Verification items for the finished model (mm, model axes). A direction names the side the tool comes from. Coordinates: 2 decimals unless noted, no trailing zeros. Loops run counter-clockwise (first coordinate to the right, second up) from the corner with the lowest first, then second, coordinate; pieces in that order, holes last.
Q1. Access from +Z, -Z, +X, -X, +Y, -Y to the whole of each face (thin tool, end or side, straight path). Record for faces 4 (the face through (21.5, -1, -2)), 5 (the face through (0.217, -2.076, -0.203)), 6 (the face through (20.7, 1.1, -1.7)), 7 (the face through (-3, 0, 8)).
Q2. Go/stop test with flat-tipped pins: P1, Ø2, axis at y = 1, z = 0.5, coming from the +X side; P2, Ø12, axis at x = 12.5, z = 13.5, coming from the +Y side; P3, Ø1.5, axis at x = 1, y = 1, coming from the -Z side. Record where each tip stops, or that it passes through.
Q3. Material ranges on probe 1 along Z at (x, y) = (1.75, -0.8); probe 2 along X at (y, z) = (-2.4, 8.25); probe 3 along X at (y, z) = (1.95, 2.75), recorded low to high.
Q4. Sectioned sample at B-B (z = 2.75). Enter the section's corners in (x, y), then the cut area to 3 significant figures.
Q5. Sectioned sample at A-A (x = 10.75). Enter the section's corners in (y, z).
Q6. Mould release check, pull along Z, two halves, no side actions. Record for faces 1 (the face through (20.74, -0.63, -1.88)), 2 (the face through (1, 0, 0)), 3 (the face through (0, 0, 16.6)): +Z half, -Z half, draft (parallel to the pull), parting line (faces both ways), or undercut.
```python
from build123d import *

# Parameters (mm, degrees)
SKETCH1_R           = 3
CASING_DEPTH        = 16.6
CASING_CHAMFER_SIZE = 0.3
SKETCH3_R           = 1
SKETCH4_R           = 0.7
EXPOSED_WIRE_DEPTH  = 1.5


with BuildPart() as part:
    # Sketch1 → Casing (new body)
    with BuildSketch(Plane.XY):
        Circle(SKETCH1_R)
    extrude(amount=CASING_DEPTH)

    # Casing Chamfer
    casing_chamfer_edges = [part.edges().sort_by_distance(p)[0] for p in [
        (-3, 0, 0),
        (-3, 0, 16.6),
    ]]
    chamfer(casing_chamfer_edges, length=CASING_CHAMFER_SIZE)

    # Wire 2: sweep along a path in Sketch2
    with BuildLine(Plane(origin=(0, 0, 0), x_dir=(1, 0, 0), z_dir=(0, 1, 0))) as wire_2_path:
        Line((0, 0), (0, 0.4))
        ThreePointArc((0, 0.4), (0.585786438, 1.814213562), (2, 2.4))
        Line((2, 2.4), (20, 2.4))
    # Sketch3 → Wire 2 (sweep)
    with BuildSketch(Plane(origin=(0, 0, 0), x_dir=(-1, 0, 0), z_dir=(0, 0, -1))):
        with Locations((0, -1.1)):
            Circle(SKETCH3_R)
        with Locations((0, 1.1)):
            Circle(SKETCH3_R)
    sweep(path=wire_2_path.line)

    # Sketch4 → Exposed Wire (add)
    with BuildSketch(Plane(origin=(20, 0, 0), x_dir=(0, 0, -1), z_dir=(1, 0, 0))):
        with Locations((2.4, 1.1)):
            Circle(SKETCH4_R)
        with Locations((2.4, -1.1)):
            Circle(SKETCH4_R)
    extrude(amount=EXPOSED_WIRE_DEPTH)


solid = part.part
```
Geometry check:
1. face 4: +Z, -Z, +X, +Y, -Y
1. face 5: none
1. face 6: +X
1. face 7: +Z
2. P1: stops at x = 3
2. P2: passes through
2. P3: stops at z = -3.39
3. probe 1: z = -3.34 to -1.42, 0 to 16.6
3. probe 2: x = -1.8 to 1.8
3. probe 3: x = -2.28 to 2.28
4. outline: circle Ø6 at (0, 0)
4. area: 28.3 mm2
5. outline: circle Ø2 at (-1.1, -2.4); circle Ø2 at (1.1, -2.4)
6. face 1: parting line
6. face 2: undercut
6. face 3: +Z half
